```python
from build123d import *

# Parameters (mm, degrees)
F0_R     = 18.75
F1_DEPTH = 15
F3_DEPTH = 3
F4_R     = 1.6
F5_DEPTH = 25
F6_R     = 3
F7_DEPTH = 7


with BuildPart() as f1:
    # F0 (on Top) → F1 (new body)
    with BuildSketch(Plane.XY):
        Circle(F0_R)
    extrude(amount=F1_DEPTH)

    # F2 (on face) → F3 (cut)
    with BuildSketch(Plane.XY.offset(15)):
        Polygon((2.875, -1.659882), (2.875, 1.659882), (0, 3.319764), (-2.875, 1.659882), (-2.875, -1.659882), (0, -3.319764), align=None)
    extrude(amount=-F3_DEPTH, mode=Mode.SUBTRACT)

    # F4 (on face) → F5 (cut)
    with BuildSketch(Plane.XY.offset(12)):
        Circle(F4_R)
    extrude(amount=-F5_DEPTH, mode=Mode.SUBTRACT)

    # F6 (on face) → F7 (cut)
    with BuildSketch(Plane.XY):
        Circle(F6_R)
    extrude(amount=F7_DEPTH, mode=Mode.SUBTRACT)


solid = f1.part
```
Model file for the job. Use its own axes, mm. A direction names the side the tool comes from. Round coordinates to 2 decimals unless told otherwise and drop trailing zeros. Write each loop counter-clockwise with the first axis right and the second up, starting at its lowest first coordinate (ties: lowest second). Pieces come first, ordered by that corner, then holes. Notation, with made-up numbers: (-19.5, 9.5) - (-1.5, 9.5) arc R16 ccw to (-1.5, 15.5) - close; hole circle Ø5 at (10.25, 55.25). An arc over 180 degrees is marked (long way). One line per item, written item: value.
(1) Cut at A-A, the plane y = 0. Give the cut face in (x, z) (3 decimals), plus the area to 3 significant figures.
Values follow:
outline: (-18.75, 0) - (-3, 0) - (-3, 7) - (-1.6, 7) - (-1.6, 12) - (-2.875, 12) - (-2.875, 15) - (-18.75, 15) - close; (1.6, 7) - (3, 7) - (3, 0) - (18.75, 0) - (18.75, 15) - (2.875, 15) - (2.875, 12) - (1.6, 12) - close
area: 487 mm²
(2) 3-axis set-ups, long thin cutter, end or side, ignore diameter. For faces 1 (the cylindrical face through (-3, 0, 3)), 2 (the flat face through (4, 0, 15)), 3 (the flat face through (1.458, 2.478, 13.521)): which of +Z, -Z, +X, -X, +Y, -Y reach the whole face in a straight line?
Values follow:
face 1: -Z
face 2: +Z, +X, -X, +Y, -Y
face 3: +Z
(3) Wall check: probe 1 along Y at (x, z) = (0, 10.65); probe 2 along Y at (x, z) = (0, 4.25); probe 3 along X at (y, z) = (-2, 5.25). Give the ranges that are in metal, low to high.
Values follow:
probe 1: y = -18.75 to -1.6, 1.6 to 18.75
probe 2: y = -18.75 to -3, 3 to 18.75
probe 3: x = -18.64 to -2.24, 2.24 to 18.64
(4) Cut at B-B, the plane z = 1.5. Give the cut face in (x, y).
Values follow:
outline: circle Ø37.5 at (0, 0); hole circle Ø6 at (0, 0)
(5) Cut at C-C, the plane x = 15. Give the cut face in (y, z).
Values follow:
outline: (-11.25, 0) - (11.25, 0) - (11.25, 15) - (-11.25, 15) - close
(6) Drop flat-ended pins along their axis: P1, Ø2, axis at y = 9.5, z = 10.5, coming from the -X side; P2, Ø5, axis at y = 7.5, z = 8, coming from the -X side; P3, Ø5, axis at x = 0, y = 0, coming from the -Z side. Give the stop position or say it passes through.
Values follow:
P1: stops at x = -16.71
P2: stops at x = -18.07
P3: stops at z = 7
(7) Cut at D-D, the plane z = 10. Give the cut face in (x, y), plus the area to 3 significant figures.
Values follow:
outline: circle Ø37.5 at (0, 0); hole circle Ø3.2 at (0, 0)
area: 1,100 mm²
